```python
from build123d import *

# Parameters (mm, degrees)
SKETCH1_W                    = 21.59
SKETCH1_H                    = 46.99
SKETCH1_R                    = 4.124999878
BOSS_EXTRUDE1_DEPTH          = 3.175
EDGE_FLANGE2_STRIP_W         = 19.05
EDGE_FLANGE2_STRIP_H         = 3.175
EDGE_FLANGE2_STRIP_CUT_DEPTH = 21.59
EDGE_FLANGE2_DEPTH           = 21.59
EDGE_FLANGE2_FLAT_DEPTH      = 3.175
EDGE_FLANGE3_STRIP_W         = 15.900000204
EDGE_FLANGE3_STRIP_H         = 3.175
EDGE_FLANGE3_STRIP_CUT_DEPTH = 19.05
EDGE_FLANGE3_DEPTH           = 19.05


# Sheet-metal steps are written as plain solids
with BuildPart() as part:
    # Sketch1 → Boss-Extrude1 (new body)
    with BuildSketch(Plane.XY):
        with Locations((10.795, 23.495)):
            Rectangle(SKETCH1_W, SKETCH1_H)
        with Locations(Location((10.795, 39.729801599, 0), (0, 0, 180))):
            Circle(SKETCH1_R, mode=Mode.SUBTRACT)
    extrude(amount=BOSS_EXTRUDE1_DEPTH)

    # Edge-Flange2 strip (across the edge) → Edge-Flange2 strip cut (cut)
    with BuildSketch(Plane(origin=(21.59, 0, 0), x_dir=(0, 1, 0), z_dir=(-1, 0, 0))):
        with Locations((-3.175, -1.5875)):
            Rectangle(EDGE_FLANGE2_STRIP_W, EDGE_FLANGE2_STRIP_H)
    extrude(amount=EDGE_FLANGE2_STRIP_CUT_DEPTH, mode=Mode.SUBTRACT)

    # Edge-Flange2 bend section (across the edge) → Edge-Flange2 (add)
    with BuildSketch(Plane(origin=(21.59, 0, 0), x_dir=(0, 1, 0), z_dir=(-1, 0, 0))):
        with BuildLine():
            Line((0, 3.175), (3.175, 3.175))
            ThreePointArc((3.175, 3.175), (4.10493597, 0.92993597), (6.35, 0))
            Line((6.35, 0), (6.35, -3.175))
            ThreePointArc((6.35, -3.175), (1.859871939, -1.315128061), (0, 3.175))
        make_face()
    extrude(amount=EDGE_FLANGE2_DEPTH)

    # Edge-Flange2 profile (on flange) → Edge-Flange2 flat (add)
    with BuildSketch(Plane(origin=(0, 0, 0), x_dir=(-1, 0, 0), z_dir=(0, -1, 0))):
        Polygon((0, 3.175), (0, 31.493260102), (27.326645128, 31.493260102), (27.326645128, 50.543260102), (0, 50.543260102), (-21.59, 50.543260102), (-21.59, 3.175), align=None)
    extrude(amount=-EDGE_FLANGE2_FLAT_DEPTH)

    # Edge-Flange3 strip (across the edge) → Edge-Flange3 strip cut (cut)
    with BuildSketch(Plane(origin=(-27.326645128, 3.175, -50.543260102), x_dir=(1, 0, 0), z_dir=(0, 0, 1))):
        with Locations((-6.35, -1.5875)):
            Rectangle(EDGE_FLANGE3_STRIP_W, EDGE_FLANGE3_STRIP_H)
    extrude(amount=EDGE_FLANGE3_STRIP_CUT_DEPTH, mode=Mode.SUBTRACT)

    # Edge-Flange3 section (across the edge) → Edge-Flange3 (add)
    with BuildSketch(Plane(origin=(-27.326645128, 3.175, -50.543260102), x_dir=(1, 0, 0), z_dir=(0, 0, 1))):
        with BuildLine():
            Line((-3.175, 1.600000102), (-3.175, 36.703))
            Line((-3.175, 36.703), (0, 36.703))
            Line((0, 36.703), (0, 1.600000102))
            ThreePointArc((0, 1.600000102), (0.46862918, 0.46862918), (1.600000102, 0))
            Line((1.600000102, 0), (1.600000102, -3.175))
            ThreePointArc((1.600000102, -3.175), (-1.77643485, -1.77643485), (-3.175, 1.600000102))
        make_face()
    extrude(amount=EDGE_FLANGE3_DEPTH)


solid = part.part
```
CAD build for the part. Positions are in the model's coordinates, mm. A direction names the side the tool comes from. Round coordinates to 2 decimals unless told otherwise and drop trailing zeros. Write each loop counter-clockwise with the first axis right and the second up, starting at its lowest first coordinate (ties: lowest second). Pieces come first, ordered by that corner, then holes. Notation, with made-up numbers: (47, 7.25) - (75, 7.25) arc R30 cw to (75, 29.25) - close; hole circle Ø6 at (50, 70.5). An arc over 180 degrees is marked (long way). Return JSON: item names as keys, results as strings. Group by question number.
Item 1: Band-saw the part on B-B on x = 12.5. List the corners of the cut face in (y, z) (3 decimals), plus the area to 3 significant figures.
Item 2: Band-saw the part on C-C on z = -43. List the corners of the cut face in (x, y) (3 decimals).
Item 3: Band-saw the part on A-A on y = 18.5. List the corners of the cut face in (x, z) (3 decimals), plus the area to 3 significant figures.
Item 4: 3-axis set-ups, long thin cutter, end or side, ignore diameter. For faces 4 (the face through (0, 15, 1)), 5 (the face through (11, 27, 0)), 6 (the face through (4, 3.175, -32)): which of +Z, -Z, +X, -X, +Y, -Y reach the whole face in a straight line?
Item 5: Band-saw the part on D-D on x = 5. List the corners of the cut face in (y, z) (3 decimals).
Item 6: Probe probe 1 along Z at (x, y) = (11, 22) (3 decimals); probe 2 along Z at (x, y) = (-28, 38). List the from-to ranges inside material, lowest first.
Item 7: Flat gauge pins, fed straight in: pin 1 Ø4 at (x, y) = (16.5, 40.5) entering from -Z; pin 2 Ø6 at (x, z) = (14, -7.5) entering from -Y; pin 3 Ø9.5 at (y, z) = (29.5, -42) entering from +X; pin 4 Ø12 at (y, z) = (35, -3) entering from -X. Where does each tip first touch, or does it go through?
Item 8: Mould opens along Y. For faces 1 (the face through (-26.87, 3.656, -41.152)), 2 (the face through (11.33, 35.64, 1.57)), 3 (the face through (11, 27, 3.175)) say: +Y half, -Y half, draft (parallel to the pull), parting line (faces both ways), or undercut.
Resolved:
{
 "1": {"outline": "(0, -50.543) - (3.175, -50.543) - (3.175, -3.175) arc R3.175 cw to (6.35, 0) - (35.974, 0) - (35.974, 3.175) - (6.35, 3.175) arc R6.35 ccw to (0, -3.175) - close; (43.486, 0) - (46.99, 0) - (46.99, 3.175) - (43.486, 3.175) - close", "area": "279 mm²"},
 "2": {"outline": "(-30.502, 4.775) arc R4.775 ccw to (-25.727, 0) - (21.59, 0) - (21.59, 3.175) - (-25.727, 3.175) arc R1.6 cw to (-27.327, 4.775) - (-27.327, 39.878) - (-30.502, 39.878) - close"},
 "3": {"outline": "(-30.502, -50.543) - (-27.327, -50.543) - (-27.327, -31.493) - (-30.502, -31.493) - close; (0, 0) - (21.59, 0) - (21.59, 3.175) - (0, 3.175) - close", "area": "129 mm²"},
 "4": {"face 4": "+Z, -X, +Y, -Y", "face 5": "-Z, +X, -X, +Y", "face 6": "-Z, +X, +Y"},
 "5": {"outline": "(0, -50.543) - (3.175, -50.543) - (3.175, -3.175) arc R3.175 cw to (6.35, 0) - (46.99, 0) - (46.99, 3.175) - (6.35, 3.175) arc R6.35 ccw to (0, -3.175) - close"},
 "6": {"probe 1": "z = 0 to 3.175", "probe 2": "z = -50.54 to -31.49"},
 "7": {"pin 1": "stops at z = 0", "pin 2": "stops at y = 0", "pin 3": "stops at x = -27.33", "pin 4": "stops at x = 0"},
 "8": {"face 1": "+Y half", "face 2": "undercut", "face 3": "draft"}
}
